Verification items for the finished model (mm, model axes). A direction names the side the tool comes from. Give positions to 0.01 mm unless a question says otherwise; leave off trailing zeros. Loops run counter-clockwise (first coordinate to the right, second up) from the corner with the lowest first, then second, coordinate; pieces in that order, holes last. Notation, with made-up numbers: M 22,18.25 L 79,18.25 A20 cw 79,57.25 Z; hole C 45.5,-23.75 d4. An arc over 180 degrees is marked long. Answer in a Markdown table with one row per item.
```python
from build123d import *

# Parameters (mm, degrees)
SKETCH1_R          = 0.79375
EXTRUDE1_DEPTH     = 6.0325
SKETCH2_W          = 9.525
SKETCH2_H          = 6.477
CUT_EXTRUDE1_DEPTH = 25.353636695
FILLET1_R          = 2.921
EXTRUDE2_DEPTH     = 12.065
SKETCH5_W          = 1.5875
SKETCH5_H          = 10.676085567
CUT_EXTRUDE2_DEPTH = 4.572


with BuildPart() as part:
    # Sketch1 → Extrude1 (new, symmetric)
    with BuildSketch(Plane(origin=(0, 0, 0), x_dir=(0, 0, -1), z_dir=(1, 0, 0))):
        with BuildLine():
            Line((0, 2.921), (22.86, 2.921))
            Line((22.86, 2.921), (22.86, -2.921))
            Line((22.86, -2.921), (0, -2.921))
            ThreePointArc((0, -2.921), (-2.921, 0), (0, 2.921))
        make_face()
        with Locations(Location((0, 0, 0), (0, 0, 180))):
            Circle(SKETCH1_R, mode=Mode.SUBTRACT)
        with Locations(Location((19.939, 0, 0), (0, 0, 180))):
            Circle(SKETCH1_R, mode=Mode.SUBTRACT)
    extrude(amount=EXTRUDE1_DEPTH, both=True)

    # Sketch2 → Cut-Extrude1 (cut, through all)
    with BuildSketch(Plane(origin=(0, 2.921, 0), x_dir=(-1, 0, 0), z_dir=(0, 1, 0))):
        with Locations((0, -0.3175)):
            Rectangle(SKETCH2_W, SKETCH2_H)
    extrude(amount=-CUT_EXTRUDE1_DEPTH, mode=Mode.SUBTRACT)

    # Fillet1
    fillet1_edges = [part.edges().sort_by_distance(p)[0] for p in [
        (0, 2.921, -22.86),
        (0, -2.921, -22.86),
    ]]
    fillet(fillet1_edges, radius=FILLET1_R - 0.0001)  # a hair under: the kernel refuses the full size

    # Sketch3 → Extrude2 (add)
    with BuildSketch(Plane(origin=(6.0325, 0, 0), x_dir=(0, 0, -1), z_dir=(1, 0, 0))):
        with BuildLine():
            Line((22.468660204, 1.4605), (24.265085567, -1.651))
            Line((24.265085567, -1.651), (24.265085567, -2.921))
            Line((24.265085567, -2.921), (19.939, -2.921))
            ThreePointArc((19.939, -2.921), (22.004458908, -2.065458908), (22.86, 0))
            ThreePointArc((22.86, 0), (22.760469339, 0.756010431), (22.468660204, 1.4605))
        make_face()
    extrude(amount=-EXTRUDE2_DEPTH)

    # Sketch5 → Cut-Extrude2 (cut)
    with BuildSketch(Plane(origin=(0, 2.921, 0), x_dir=(-1, 0, 0), z_dir=(0, 1, 0))):
        with Locations((0, -18.927042783)):
            Rectangle(SKETCH5_W, SKETCH5_H)
    extrude(amount=-CUT_EXTRUDE2_DEPTH, mode=Mode.SUBTRACT)


solid = part.part
```
Item 1: Sectioned sample at B-B (y = 0). Record the cut outline in (x, z).
Reported:
| item | result |
|---|---|
| outline | M -6.03,-23.31 L -0.79,-23.31 L -0.79,-20.73 L -6.03,-20.73 Z; M -6.03,-19.15 L -0.79,-19.15 L -0.79,-13.59 L 0.79,-13.59 L 0.79,-19.15 L 6.03,-19.15 L 6.03,-0.79 L 4.76,-0.79 L 4.76,-3.56 L -4.76,-3.56 L -4.76,-0.79 L -6.03,-0.79 Z; M -6.03,0.79 L -4.76,0.79 L -4.76,2.92 L -6.03,2.92 Z; M 0.79,-23.31 L 6.03,-23.31 L 6.03,-20.73 L 0.79,-20.73 Z; M 4.76,0.79 L 6.03,0.79 L 6.03,2.92 L 4.76,2.92 Z |
Item 2: Release check for a two-part mould opening along Y. For faces 1 (the cylindrical face through (5.41, -0.06, 2.92)), 2 (the cylindrical face through (-5.41, 0.7, 0.37)), 3 (the flat face through (0, -2.921, -12)) record: released by +Y, released by -Y, zero draft, split by the parting line, or undercut.
Reported:
| item | result |
|---|---|
| face 1 | split by the parting line |
| face 2 | undercut |
| face 3 | released by -Y |
Item 3: Tool access check on faces 4 (the flat face through (4.762, 0, -1)), 5 (the flat face through (6.032, 0, -11)), 6 (the flat face through (0, -1.651, -19)). Record the directions out of +Z, -Z, +X, -X, +Y, -Y that give a thin tool (end or side, any length) a straight path to the whole face; none if there is none.
Reported:
| item | result |
|---|---|
| face 4 | +Z, +Y, -Y |
| face 5 | +Z, -Z, +X, +Y, -Y |
| face 6 | -Z, +Y |
Item 4: Scan lines: L1, parallel to X at y = -0.1, z = -2.25; L2, parallel to Z at x = -4, y = -0.35; L3, parallel to Z at x = -0.75, y = 0.1. Record each from-to range of solid material in increasing order. Write a range as [from, to].
Reported:
| item | result |
|---|---|
| L1 | x = [-6.03, -4.76], [4.76, 6.03] |
| L2 | z = [-23.51, -20.65], [-19.23, -3.56] |
| L3 | z = [-13.59, -3.56] |
Item 5: Sectioned sample at D-D (y = 2.15). Record the cut outline in (x, z).
Reported:
| item | result |
|---|---|
| outline | M -6.03,-21.92 L -0.79,-21.92 L -0.79,-13.59 L 0.79,-13.59 L 0.79,-21.92 L 6.03,-21.92 L 6.03,1.98 L 4.76,1.98 L 4.76,-3.56 L -4.76,-3.56 L -4.76,1.98 L -6.03,1.98 Z |
Item 6: Go/stop test with flat-tipped pins: pin 1 (1.4 mm diameter, centred on y = 0, z = -19.939, fed in from -X); pin 2 (1 mm diameter, centred on x = -3, y = 0, fed in from -Z); pin 3 (1.3 mm diameter, centred on x = 0, z = -21, fed in from +Y); pin 4 (1.5 mm diameter, centred on x = -3.5, y = 0, fed in from -Z). Record where each tip stops, or that it passes through.
Reported:
| item | result |
|---|---|
| pin 1 | passes through |
| pin 2 | stops at z = -23.6 |
| pin 3 | stops at y = -1.65 |
| pin 4 | stops at z = -23.74 |
Item 7: Sectioned sample at C-C (z = -20.25). Record the cut outline in (x, y).
Reported:
| item | result |
|---|---|
| outline | M -6.03,-2.92 L 6.03,-2.92 L 6.03,-0.73 L 0.79,-0.73 L 0.79,-1.65 L -0.79,-1.65 L -0.79,-0.73 L -6.03,-0.73 Z; M -6.03,0.73 L -0.79,0.73 L -0.79,2.9 L -6.03,2.9 Z; M 0.79,0.73 L 6.03,0.73 L 6.03,2.9 L 0.79,2.9 Z |
Item 8: Sectioned sample at A-A (x = 4.5). Record the cut outline in (y, z), and give its area (3 significant figures).
Reported:
| item | result |
|---|---|
| outline | M -2.92,-24.27 L -1.65,-24.27 L 1.45,-22.48 A2.92 ccw 2.92,-19.94 L 2.92,-3.56 L -2.92,-3.56 Z; hole C 0,-19.94 d1.59 |
| area | 113 mm^2 |
